Verification items for the finished model (mm, model axes). Face numbers are marked on the shaded views. Round coordinates to 2 decimals unless told otherwise and drop trailing zeros. Loops run counter-clockwise (first coordinate to the right, second up) from the corner with the lowest first, then second, coordinate; pieces in that order, holes last. Notation, with made-up numbers: (-20.5, 2.25) -> (31.5, 2.25) arc R21 cw to (31.5, 37.25) -> close; hole circle Ø3 at (-23.75, -17). An arc over 180 degrees is marked (long way). Write item = value, one per line.
```python
from build123d import *

# Parameters (mm, degrees)
SKETCH1_R           = 16.4
SKETCH1_R_2         = 11.4
BOSS_EXTRUDE1_DEPTH = 95
BOSS_EXTRUDE2_START = 5
BOSS_EXTRUDE2_DEPTH = 5
CUT_EXTRUDE1_START  = -5
CUT_EXTRUDE1_DEPTH  = 5


with BuildPart() as part:
    # Sketch1 → Boss-Extrude1 (new body)
    with BuildSketch(Plane.XY):
        Circle(SKETCH1_R)
        Circle(SKETCH1_R_2, mode=Mode.SUBTRACT)
    extrude(amount=BOSS_EXTRUDE1_DEPTH)

    # Sketch3 → Boss-Extrude2 (add)
    with BuildSketch(Plane(origin=(0, 0, 0), x_dir=(-1, 0, 0), z_dir=(0, 0, -1)).offset(BOSS_EXTRUDE2_START)):
        with BuildLine():
            Line((13.164725595, 2.5), (16.208331191, 2.5))
            ThreePointArc((16.208331191, 2.5), (16.4, 0), (16.208331191, -2.5))
            Line((16.208331191, -2.5), (13.164725595, -2.5))
            ThreePointArc((13.164725595, -2.5), (13.4, 0), (13.164725595, 2.5))
        make_face()
        with BuildLine():
            Line((-16.208331191, 2.5), (-13.164725595, 2.5))
            ThreePointArc((-13.164725595, 2.5), (-13.4, 0), (-13.164725595, -2.5))
            Line((-13.164725595, -2.5), (-16.208331191, -2.5))
            ThreePointArc((-16.208331191, -2.5), (-16.4, 0), (-16.208331191, 2.5))
        make_face()
    extrude(amount=-BOSS_EXTRUDE2_DEPTH)

    # Sketch4 → Cut-Extrude1 (cut)
    with BuildSketch(Plane.XY.offset(95).offset(CUT_EXTRUDE1_START)):
        with BuildLine():
            Line((13.164725595, 2.5), (16.208331191, 2.5))
            ThreePointArc((16.208331191, 2.5), (16.4, 0), (16.208331191, -2.5))
            Line((16.208331191, -2.5), (13.164725595, -2.5))
            ThreePointArc((13.164725595, -2.5), (13.4, 0), (13.164725595, 2.5))
        make_face()
        with BuildLine():
            Line((-16.208331191, 2.5), (-13.164725595, 2.5))
            ThreePointArc((-13.164725595, 2.5), (-13.4, 0), (-13.164725595, -2.5))
            Line((-13.164725595, -2.5), (-16.208331191, -2.5))
            ThreePointArc((-16.208331191, -2.5), (-16.4, 0), (-16.208331191, 2.5))
        make_face()
    extrude(amount=CUT_EXTRUDE1_DEPTH, mode=Mode.SUBTRACT)


solid = part.part
```
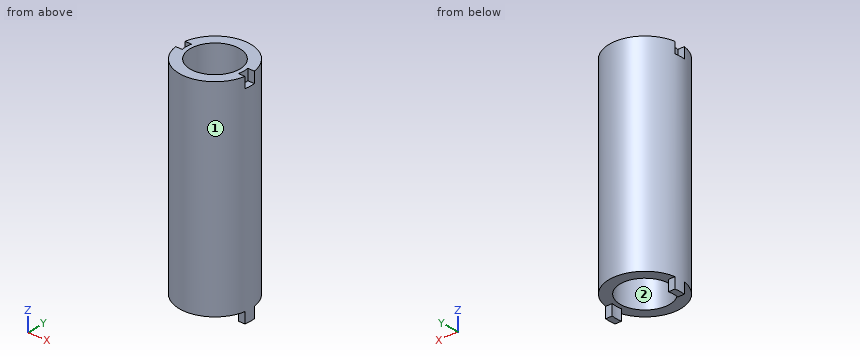
(1) Material ranges on probe 1 along Y at (x, z) = (0, 55); probe 2 along Y at (x, z) = (-4, 64); probe 3 along Z at (x, y) = (12.5, 3), recorded low to high. Write a range as from..to.
Filled sheet:
probe_1 = -16.4..-11.4, 11.4..16.4
probe_2 = -15.9..-10.68, 10.68..15.9
probe_3 = 0..95
(2) Sectioned sample at A-A, the plane y = 0. Record the cut outline in (x, z).
Filled sheet:
outline = (-16.4, -5) -> (-13.4, -5) -> (-13.4, 0) -> (-11.4, 0) -> (-11.4, 95) -> (-13.4, 95) -> (-13.4, 90) -> (-16.4, 90) -> close; (11.4, 0) -> (13.4, 0) -> (13.4, -5) -> (16.4, -5) -> (16.4, 90) -> (13.4, 90) -> (13.4, 95) -> (11.4, 95) -> close
(3) Draft check along X on the marked faces 1 and 2. Enter one of: released by +X, released by -X, zero draft, split by the parting line, or undercut.
Filled sheet:
face_1 = split by the parting line
face_2 = undercut
(4) Go/stop test with flat-tipped pins: pin 1 Ø3.5 at (x, z) = (-15.5, 91.5) entering from +Y; pin 2 Ø12 at (y, z) = (9.5, 72.5) entering from +X; pin 3 Ø1.6 at (x, y) = (-14.5, -1) entering from +Z. Record where each tip stops, or that it passes through.
Filled sheet:
pin_1 = 8.94
pin_2 = 16.02
pin_3 = 90
(5) Sectioned sample at D-D, the plane x = -5. Record the cut outline in (y, z) (3 decimals), and give its area (3 significant figures).
Filled sheet:
outline = (-15.619, 0) -> (-10.245, 0) -> (-10.245, 95) -> (-15.619, 95) -> close; (10.245, 0) -> (15.619, 0) -> (15.619, 95) -> (10.245, 95) -> close
area = 1,020 mm2
(6) Sectioned sample at B-B, the plane x = 0. Record the cut outline in (y, z), and give its area (3 significant figures).
Filled sheet:
outline = (-16.4, 0) -> (-11.4, 0) -> (-11.4, 95) -> (-16.4, 95) -> close; (11.4, 0) -> (16.4, 0) -> (16.4, 95) -> (11.4, 95) -> close
area = 950 mm2
(7) Sectioned sample at C-C, the plane z = 18. Record the cut outline in (x, y), and give its area (3 significant figures).
Filled sheet:
outline = circle Ø32.8 at (0, 0); hole circle Ø22.8 at (0, 0)
area = 437 mm2
